Work out the finished part from the listing and answer in its coordinate system (mm). A direction names the side the tool comes from. Coordinates: 2 decimals unless noted, no trailing zeros. Write each loop counter-clockwise with the first axis right and the second up, starting at its lowest first coordinate (ties: lowest second). Pieces come first, ordered by that corner, then holes. Notation, with made-up numbers: M 64.5,75 L 85.5,75 A19 ccw 85.5,106 Z; hole C 11,-27.75 d7. An arc over 180 degrees is marked long. Use CSV: the item, a comma, the result in double quotes.
from build123d import *

# Parameters (mm, degrees)
F1_DEPTH = 30
F2_W     = 11
F2_H     = 15
F3_DEPTH = 11
F4_W     = 15
F4_H     = 8
F5_DEPTH = 11
F6_ANGLE = -90


with BuildPart() as f1:
    # F0 (on Front) → F1 (new body)
    with BuildSketch(Plane.XZ):
        Polygon((0, 30), (0, 0), (40, 0), (40, 11), (11, 11), (11, 30), align=None)
    extrude(amount=F1_DEPTH)

    # F2 (on face) → F3 (cut, through all)
    with BuildSketch(Plane.XY.offset(11)):
        with Locations((34.5, -22.5)):
            Rectangle(F2_W, F2_H)
    extrude(amount=-F3_DEPTH, mode=Mode.SUBTRACT)

    # F4 (on face) → F5 (cut, through all)
    with BuildSketch(Plane.YZ.offset(11)):
        with Locations((-22.5, 26)):
            Rectangle(F4_W, F4_H)
    extrude(amount=-F5_DEPTH, mode=Mode.SUBTRACT)


with BuildPart() as f1_1:
    # F6: moved
    add(f1.part.rotate(Axis((0, 0, 15), (0, 0, 1)), F6_ANGLE))


solid = f1_1.part
Item 1: The part is cut by section D-D (z = 26.5). Write down the section's boundary in (x, y), then the cut area to 3 significant figures.
Answer:
outline,"M -15,-11 L 0,-11 L 0,0 L -15,0 Z"
area,"165 mm2"
Item 2: The part is cut by section C-C (z = 12.5). Write down the section's boundary in (x, y), then the cut area to 3 significant figures.
Answer:
outline,"M -30,-11 L 0,-11 L 0,0 L -30,0 Z"
area,"330 mm2"
Item 3: A tool of negligible diameter and unlimited length cuts with its end or side. For faces 1 (the face through (-23, -29, 6)), 2 (the face through (-15, -22, 11)), 3 (the face through (-15, -6, 26)), from which of +Z, -Z, +X, -X, +Y, -Y can it reach the whole face along a straight path? Write none if from no direction.
Answer:
face 1,"+Z, -Z, -X, -Y"
face 2,"+Z, +X, -X, -Y"
face 3,"+Z, -X, +Y, -Y"
Item 4: Consider probe 1 along Z at (x, y) = (-19, -8); probe 2 along Z at (x, y) = (-10.5, -15); probe 3 along Y at (x, z) = (-28, 4). Determine where each line is inside the solid, lowest interval first.
Answer:
probe 1,"z = 0 to 22"
probe 2,"z = 0 to 11"
probe 3,"y = -29 to 0"
Item 5: The part is cut by section A-A (y = -4.5). Write down the section's boundary in (x, z), then the cut area to 3 significant figures.
Answer:
outline,"M -30,0 L 0,0 L 0,30 L -15,30 L -15,22 L -30,22 Z"
area,"780 mm2"
Item 6: The part is cut by section B-B (x = -3). Write down the section's boundary in (y, z), then the cut area to 3 significant figures.
Answer:
outline,"M -40,0 L 0,0 L 0,30 L -11,30 L -11,11 L -40,11 Z"
area,"649 mm2"
Item 7: Given pin 1 (2.5 mm diameter, centred on y = -6.5, z = 26.5, fed in from -X); pin 2 (12 mm diameter, centred on x = -23, y = -7, fed in from +Z); pin 3 (12 mm diameter, centred on x = -22, z = 6, fed in from -Y); pin 4 (12 mm diameter, centred on y = -33.5, z = 4, fed in from -X), each flat-ended and moving along its own axis, determine where each tip first touches the part or whether it passes through.
Answer:
pin 1,"stops at x = -15"
pin 2,"stops at z = 22"
pin 3,"stops at y = -29"
pin 4,"stops at x = -30"
